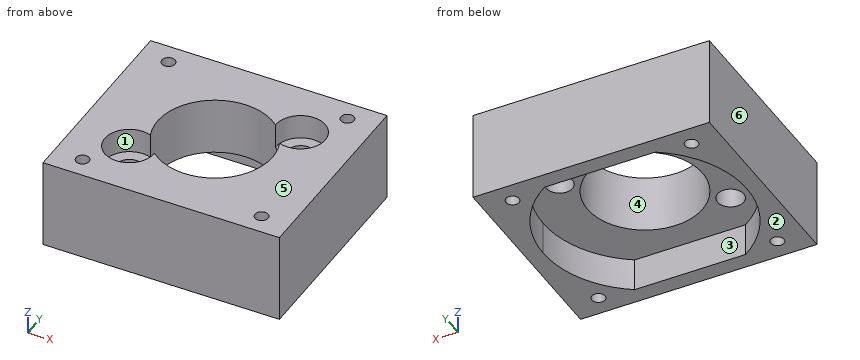
```python
from build123d import *

# Parameters (mm, degrees)
SKETCH_1_W          = 14.4
SKETCH_1_H          = 12.4
EXTRUDE_1_DEPTH     = 3.5
SKETCH_3_R          = 0.8
SKETCH_3_R_2        = 3.5
CUT_EXTRUDE_1_DEPTH = 11.125709852
SKETCH_3_3_R        = 1.5
CUT_EXTRUDE_2_DEPTH = 1.5
EXTRUDE_2_DEPTH     = 2
SKETCH_5_R          = 0.4
CUT_EXTRUDE_3_DEPTH = 11.978615578


with BuildPart() as part:
    # 草图1 → 凸台-拉伸1 (new body)
    with BuildSketch(Plane.XY):
        Rectangle(SKETCH_1_W, SKETCH_1_H)
    extrude(amount=EXTRUDE_1_DEPTH)

    # 草图3 → 切除-拉伸1 (cut, through all)
    with BuildSketch(Plane.XY.offset(3.5)):
        with Locations((3.785828839, 2.7)):
            Circle(SKETCH_3_R)
        with Locations((-3.785828839, -2.7)):
            Circle(SKETCH_3_R)
        Circle(SKETCH_3_R_2)
    extrude(amount=-CUT_EXTRUDE_1_DEPTH, mode=Mode.SUBTRACT)

    # 草图3<3> → 切除-拉伸2 (cut)
    with BuildSketch(Plane.XY.offset(3.5)):
        with Locations((3.785828839, 2.7)):
            Circle(SKETCH_3_3_R)
        with Locations((-3.785828839, -2.7)):
            Circle(SKETCH_3_3_R)
    extrude(amount=-CUT_EXTRUDE_2_DEPTH, mode=Mode.SUBTRACT)

    # 草图4 → 凸台-拉伸2 (add)
    with BuildSketch(Plane(origin=(0, 0, 0), x_dir=(-1, 0, 0), z_dir=(0, 0, -1))):
        with BuildLine():
            Line((-6.2, 0), (-6.2, 5.2))
            Line((-6.2, 5.2), (-3.376388603, 5.2))
            ThreePointArc((-3.376388603, 5.2), (-1.760681692, 5.944745577), (-1.3e-08, 6.2))
            Line((-1.3e-08, 6.2), (-7.2, 6.2))
            Line((-7.2, 6.2), (-7.2, -6.2))
            Line((-7.2, -6.2), (0, -6.2))
            ThreePointArc((0, -6.2), (-1.760681686, -5.944745579), (-3.376388603, -5.2))
            Line((-3.376388603, -5.2), (-6.2, -5.2))
            Line((-6.2, -5.2), (-6.2, 0))
        make_face()
        with BuildLine():
            ThreePointArc((-1.3e-08, 6.2), (1.76068168, 5.944745581), (3.376388603, 5.2))
            Line((3.376388603, 5.2), (6.2, 5.2))
            Line((6.2, 5.2), (6.2, 0))
            Line((6.2, 0), (6.2, -5.2))
            Line((6.2, -5.2), (3.376388603, -5.2))
            ThreePointArc((3.376388603, -5.2), (1.760681686, -5.944745579), (0, -6.2))
            Line((0, -6.2), (7.2, -6.2))
            Line((7.2, -6.2), (7.2, 6.2))
            Line((7.2, 6.2), (-1.3e-08, 6.2))
        make_face()
        with BuildLine():
            Line((3.376388603, -5.2), (-3.376388603, -5.2))
            ThreePointArc((-3.376388603, -5.2), (-1.760681686, -5.944745579), (0, -6.2))
            ThreePointArc((0, -6.2), (1.760681686, -5.944745579), (3.376388603, -5.2))
        make_face()
        with BuildLine():
            ThreePointArc((-3.376388603, -5.2), (-5.448559871, -2.958579952), (-6.2, 0))
            Line((-6.2, 0), (-6.2, -5.2))
            Line((-6.2, -5.2), (-3.376388603, -5.2))
        make_face()
        with BuildLine():
            Line((-3.376388603, 5.2), (-6.2, 5.2))
            Line((-6.2, 5.2), (-6.2, 0))
            ThreePointArc((-6.2, 0), (-5.448559871, 2.958579952), (-3.376388603, 5.2))
        make_face()
        with BuildLine():
            ThreePointArc((-1.3e-08, 6.2), (-1.760681692, 5.944745577), (-3.376388603, 5.2))
            Line((-3.376388603, 5.2), (3.376388603, 5.2))
            ThreePointArc((3.376388603, 5.2), (1.76068168, 5.944745581), (-1.3e-08, 6.2))
        make_face()
        with BuildLine():
            Line((6.2, 5.2), (3.376388603, 5.2))
            ThreePointArc((3.376388603, 5.2), (5.448559871, 2.958579952), (6.2, 0))
            Line((6.2, 0), (6.2, 5.2))
        make_face()
        with BuildLine():
            Line((6.2, -5.2), (6.2, 0))
            ThreePointArc((6.2, 0), (5.448559871, -2.958579952), (3.376388603, -5.2))
            Line((3.376388603, -5.2), (6.2, -5.2))
        make_face()
    extrude(amount=EXTRUDE_2_DEPTH)

    # 草图5 → 切除-拉伸3 (cut, through all)
    with BuildSketch(Plane.XY.offset(3.5)):
        with Locations((-5.45, 4.95)):
            Circle(SKETCH_5_R)
        with Locations((5.45, 4.95)):
            Circle(SKETCH_5_R)
        with Locations((5.45, -4.95)):
            Circle(SKETCH_5_R)
        with Locations((-5.45, -4.95)):
            Circle(SKETCH_5_R)
    extrude(amount=-CUT_EXTRUDE_3_DEPTH, mode=Mode.SUBTRACT)


solid = part.part
```
Build history of the part. All positions in model axes, mm. Face numbers are marked on the shaded views. A direction names the side the tool comes from. Coordinates: 2 decimals unless noted, no trailing zeros. Order: outer loops, then holes, each group sorted by start corner. A loop starts at its lowest first (then second) coordinate and runs counter-clockwise, first axis right, second up. Notation, with made-up numbers: (62.25, 25) -> (78.25, 25) arc R20 ccw to (78.25, 55) -> close; hole circle Ø1 at (62.25, -18.5). An arc over 180 degrees is marked (long way). Answer in a Markdown table with one row per item. Add a question column.
Q1. Mould opens along X. For the marked faces 4, 5 and 6 say: +X half, -X half, draft (parallel to the pull), parting line (faces both ways), or undercut.
Q2. Band-saw the part on D-D, the plane y = -3.75. List the corners of the cut face in (x, z).
Q3. Wall check: line 1 along Y through (x, z) = (-2, -1.25); line 2 along Z through (x, y) = (5.25, 2); line 3 along X through (y, z) = (-2.25, 1.6). Give the ranges that are in metal, low to high. Write a range as [from, to].
Q4. Band-saw the part on C-C, the plane y = 4.95. List the corners of the cut face in (x, z), then the cut area to 3 significant figures.
Q5. Band-saw the part on A-A, the plane z = 0.3. List the corners of the cut face in (x, y).
Q6. Which spindle directions (+Z, -Z, +X, -X, +Y, -Y) get a long thin tool onto all of the face, cutting with end or side? Do the marked faces 1, 2 and 3. Say none if no direction does.
Q7. Drop flat-ended pins along their axis: pin 1 (2.5 mm diameter, centred on x = -3, y = -3.5, fed in from +Z); pin 2 (1.8 mm diameter, centred on x = 3.79, y = 2.7, fed in from +Z); pin 3 (1 mm diameter, centred on x = -3.5, y = -3, fed in from -Z). Give the stop position or say it passes through.
Q8. Band-saw the part on B-B, the plane x = 5.45. List the corners of the cut face in (y, z), then the cut area to 3 significant figures.
Answers follow:
| question | item | result |
|---|---|---|
| 1 | face 4 | undercut |
| 1 | face 5 | draft |
| 1 | face 6 | -X half |
| 2 | outline | (-7.2, -2) -> (-4.94, -2) -> (-4.94, 0) -> (4.94, 0) -> (4.94, -2) -> (7.2, -2) -> (7.2, 3.5) -> (-2.71, 3.5) -> (-2.71, 2) -> (-4.86, 2) -> (-4.86, 3.5) -> (-7.2, 3.5) -> close |
| 3 | line 1 | [-6.2, -5.2], [5.2, 6.2] |
| 3 | line 2 | [0, 3.5] |
| 3 | line 3 | [-7.2, -4.45], [-3.12, -2.68], [2.68, 7.2] |
| 4 | outline | (-7.2, -2) -> (-5.85, -2) -> (-5.85, 3.5) -> (-7.2, 3.5) -> close; (-5.05, -2) -> (-3.73, -2) -> (-3.73, 0) -> (3.73, 0) -> (3.73, -2) -> (5.05, -2) -> (5.05, 3.5) -> (-5.05, 3.5) -> close; (5.85, -2) -> (7.2, -2) -> (7.2, 3.5) -> (5.85, 3.5) -> close |
| 4 | area | 55.5 mm^2 |
| 5 | outline | (-7.2, -6.2) -> (7.2, -6.2) -> (7.2, 6.2) -> (-7.2, 6.2) -> close; hole circle Ø0.8 at (-5.45, -4.95); hole circle Ø0.8 at (-5.45, 4.95); hole circle Ø1.6 at (-3.79, -2.7); hole circle Ø7 at (0, 0); hole circle Ø1.6 at (3.79, 2.7); hole circle Ø0.8 at (5.45, -4.95); hole circle Ø0.8 at (5.45, 4.95) |
| 6 | face 1 | +Z |
| 6 | face 2 | -Z, +X, -X, +Y, -Y |
| 6 | face 3 | -Z |
| 7 | pin 1 | z = 3.5 |
| 7 | pin 2 | z = 2 |
| 7 | pin 3 | z = 0 |
| 8 | outline | (-6.2, -2) -> (-5.35, -2) -> (-5.35, 3.5) -> (-6.2, 3.5) -> close; (-4.55, -2) -> (-2.96, -2) -> (-2.96, 0) -> (2.96, 0) -> (2.96, -2) -> (4.55, -2) -> (4.55, 3.5) -> (-4.55, 3.5) -> close; (5.35, -2) -> (6.2, -2) -> (6.2, 3.5) -> (5.35, 3.5) -> close |
| 8 | area | 47.6 mm^2 |
